```python
from build123d import *

# Parameters (mm, degrees)
CROQUIS1_W                   = 1680
CROQUIS1_H                   = 1680
CROQUIS1_W_2                 = 1500
CROQUIS1_H_2                 = 1500
CROQUIS1_H_3                 = 90
SALIENTE_EXTRUIR1_DEPTH      = 90
TALADRO_DE_MARGEN_PARA_M61_D = 6.4


with BuildPart() as part:
    # Croquis1 → Saliente-Extruir1 (new body)
    with BuildSketch(Plane.XY):
        Rectangle(CROQUIS1_W, CROQUIS1_H)
        Rectangle(CROQUIS1_W_2, CROQUIS1_H_2, mode=Mode.SUBTRACT)
        with Locations((0, 470)):
            Rectangle(CROQUIS1_W_2, CROQUIS1_H_3)
        Polygon((-750, 55), (-750, -35), (-574.463517844, -35), (-470.54046939, -35), (470.54046939, -35), (574.463517844, -35), (750, -35), (750, 55), align=None)
        Polygon((-750, -435), (-750, -525), (750, -525), (750, -435), (343.523410168, -435), (239.600361714, -435), (-239.600361714, -435), (-343.523410168, -435), align=None)
        Polygon((-574.463517844, -35), (-343.523410168, -435), (-239.600361714, -435), (-470.54046939, -35), align=None)
        Polygon((239.600361714, -435), (343.523410168, -435), (574.463517844, -35), (470.54046939, -35), align=None)
    extrude(amount=SALIENTE_EXTRUIR1_DEPTH)

    # Taladro de margen para M61 (through all)
    with Locations(Plane.XY.offset(90)):
        with Locations((-26, 492.5), (26, 492.5), (26, 447.5), (-26, 447.5), (439.517511364, -223.733339502), (413.517511364, -268.766660498), (374.546368194, -246.266660498), (400.546368194, -201.233339502), (-413.517511364, -268.766660498), (-439.517511364, -223.733339502), (-400.546368194, -201.233339502), (-374.546368194, -246.266660498), (0, 0)):
            Hole(TALADRO_DE_MARGEN_PARA_M61_D / 2)


solid = part.part
```
The listing builds one solid part. Answer for the finished solid, in the listing's coordinates (mm). A direction names the side the tool comes from. Coordinates: 2 decimals unless noted, no trailing zeros. Loops run counter-clockwise (first coordinate to the right, second up) from the corner with the lowest first, then second, coordinate; pieces in that order, holes last. Notation, with made-up numbers: (14, -13) -> (62, -13) arc R9 cw to (62, 0) -> close; hole circle Ø8 at (-28, 19). An arc over 180 degrees is marked (long way). Use one line per item in the form item = value. Start each with the question number.
Item 1: The part is cut by section B-B on x = -88. Determine the outline of the cut face in (y, z), then the cut area to 3 significant figures.
Item 2: The part is cut by section D-D on z = 30. Count the separate pieces of the cut face and the enclosed holes in it, then the cut area to 3 significant figures.
Item 3: The mould has two halves that part along Y. Classify faces 3 (the face through (-840, -12, 44)), 4 (the face through (-12, 840, 44)), 5 (the face through (-750, 237, 44)): released by +Y, released by -Y, zero draft, split by the parting line, or undercut.
Item 4: Consider L1, parallel to Y at x = 161.5, z = 45.5; L2, parallel to X at y = 447.5, z = 33.5; L3, parallel to X at y = 674, z = 55. Determine where each line is inside the solid, lowest interval first. Write a range as [from, to].
Item 5: The part is cut by section C-C on y = -365.5. Determine the outline of the cut face in (x, z).
Item 6: A tool of negligible diameter and unlimited length cuts with its end or side. For faces 1 (the face through (840, -12, 44)), 2 (the face through (-544, -435, 44)), from which of +Z, -Z, +X, -X, +Y, -Y can it reach the whole face along a straight path? Write none if from no direction.
Item 7: The part is cut by section A-A on y = 272. Determine the outline of the cut face in (x, z).
Item 8: A flat-ended cylindrical pin translates along its axis: pin 1 Ø5 at (x, y) = (-26, 447.5) entering from +Z. Find the tip coordinate at first contact, or state that the pin passes through.
Answer key:
q1.outline = (-840, 0) -> (-750, 0) -> (-750, 90) -> (-840, 90) -> close; (-525, 0) -> (-435, 0) -> (-435, 90) -> (-525, 90) -> close; (-35, 0) -> (55, 0) -> (55, 90) -> (-35, 90) -> close; (425, 0) -> (515, 0) -> (515, 90) -> (425, 90) -> close; (750, 0) -> (840, 0) -> (840, 90) -> (750, 90) -> close
q1.area = 40,500 mm2
q2.separate_pieces = 1
q2.enclosed_holes = 19
q2.area = 1,060,000 mm2
q3.face_3 = zero draft
q3.face_4 = released by +Y
q3.face_5 = undercut
q4.L1 = [-840, -750], [-525, -435], [-35, 55], [425, 515], [750, 840]
q4.L2 = [-840, -29.2], [-22.8, 22.8], [29.2, 840]
q4.L3 = [-840, -750], [750, 840]
q5.outline = (-840, 0) -> (-750, 0) -> (-750, 90) -> (-840, 90) -> close; (-383.65, 0) -> (-279.73, 0) -> (-279.73, 90) -> (-383.65, 90) -> close; (279.73, 0) -> (383.65, 0) -> (383.65, 90) -> (279.73, 90) -> close; (750, 0) -> (840, 0) -> (840, 90) -> (750, 90) -> close
q6.face_1 = +Z, -Z, +X, +Y, -Y
q6.face_2 = +Z, -Z
q7.outline = (-840, 0) -> (-750, 0) -> (-750, 90) -> (-840, 90) -> close; (750, 0) -> (840, 0) -> (840, 90) -> (750, 90) -> close
q8.pin_1 = through
